from build123d import *

# Parameters (mm, degrees)
SKETCH1_R           = 5
BOSS_EXTRUDE1_DEPTH = 15.9
SKETCH2_R           = 11
BOSS_EXTRUDE2_DEPTH = 2


with BuildPart() as part:
    # Sketch1 → Boss-Extrude1 (new, symmetric)
    with BuildSketch(Plane(origin=(0, 0, 0), x_dir=(0, 0, -1), z_dir=(1, 0, 0))):
        Circle(SKETCH1_R)
    extrude(amount=BOSS_EXTRUDE1_DEPTH, both=True)

    # Sketch2 → Boss-Extrude2 (add)
    with BuildSketch(Plane(origin=(15.9, 0, 0), x_dir=(0, 0, -1), z_dir=(1, 0, 0))):
        Circle(SKETCH2_R)
    boss_extrude2 = extrude(amount=-BOSS_EXTRUDE2_DEPTH)

    # Mirror1: Boss-Extrude2 across plane
    add(boss_extrude2.mirror(Plane(origin=(0, 0, 0), x_dir=(0, 0, 1), z_dir=(1, 0, 0))))


solid = part.part
Here's how the part is built. I have some questions about the finished solid (model axes, mm). A direction names the side the tool comes from. Round coordinates to 2 decimals unless told otherwise and drop trailing zeros. Order: outer loops, then holes, each group sorted by start corner. A loop starts at its lowest first (then second) coordinate and runs counter-clockwise, first axis right, second up. Notation, with made-up numbers: M -30.5,-6 L -24.5,-6 A10 ccw -24.5,3 Z; hole C 21,67.5 d6. An arc over 180 degrees is marked long. One line per question, with ' | ' between items.
1) I need wall thicknesses on line 1 (X direction, y = -3, z = 6.25); line 2 (Z direction, x = 1.5, y = 0.25); line 3 (Z direction, x = -9, y = 2.5). Which ranges of each line are inside material? Lowest first, please.
Checked values:
line 1: x = -15.9 to -13.9, 13.9 to 15.9 | line 2: z = -4.99 to 4.99 | line 3: z = -4.33 to 4.33
2) Imagine slicing it at A-A, the plane z = 6. Write out the boundary of the cut face in (x, y), plus the area to 3 significant figures.
Checked values:
outline: M -15.9,-9.22 L -13.9,-9.22 L -13.9,9.22 L -15.9,9.22 Z; M 13.9,-9.22 L 15.9,-9.22 L 15.9,9.22 L 13.9,9.22 Z | area: 73.8 mm²
3) We'd pull the mould along X, two halves only. Please class faces 1 (the flat face through (15.9, 0, 0)), 2 (the flat face through (-15.9, 0, 0)), 3 (the cylindrical face through (0.19, -4.88, 1.08)), 4 (the flat face through (-13.9, -5, -2)): released by +X, released by -X, zero draft, split by the parting line, or undercut.
Checked values:
face 1: released by +X | face 2: released by -X | face 3: undercut | face 4: undercut
4) Imagine slicing it at C-C, the plane y = 0. Write out the boundary of the cut face in (x, z), plus the area to 3 significant figures.
Checked values:
outline: M -15.9,-11 L -13.9,-11 L -13.9,-5 L 13.9,-5 L 13.9,-11 L 15.9,-11 L 15.9,11 L 13.9,11 L 13.9,5 L -13.9,5 L -13.9,11 L -15.9,11 Z | area: 366 mm²
5) I'm going to push flat-ended pins straight in: pin 1 Ø6 at (x, y) = (1, -7.5) entering from -Z; pin 2 Ø12 at (x, y) = (-4, -5) entering from -Z; pin 3 Ø1.5 at (x, y) = (-4, 7) entering from -Z; pin 4 Ø1 at (x, y) = (11.5, 4.5) entering from -Z. Where does each tip first touch, or does it pass through?
Checked values:
pin 1: stops at z = -2.18 | pin 2: stops at z = -5 | pin 3: passes through | pin 4: stops at z = -3
6) On a 3-axis mill with a long thin cutter (end or side, diameter ignored), from which of +Z, -Z, +X, -X, +Y, -Y can I reach the whole of each face in a straight line? I mean faces 5 (the cylindrical face through (-14.91, -10.74, 2.38)), 6 (the flat face through (13.9, -5, -2)). Say none if no direction works.
Checked values:
face 5: +X, -X | face 6: none
